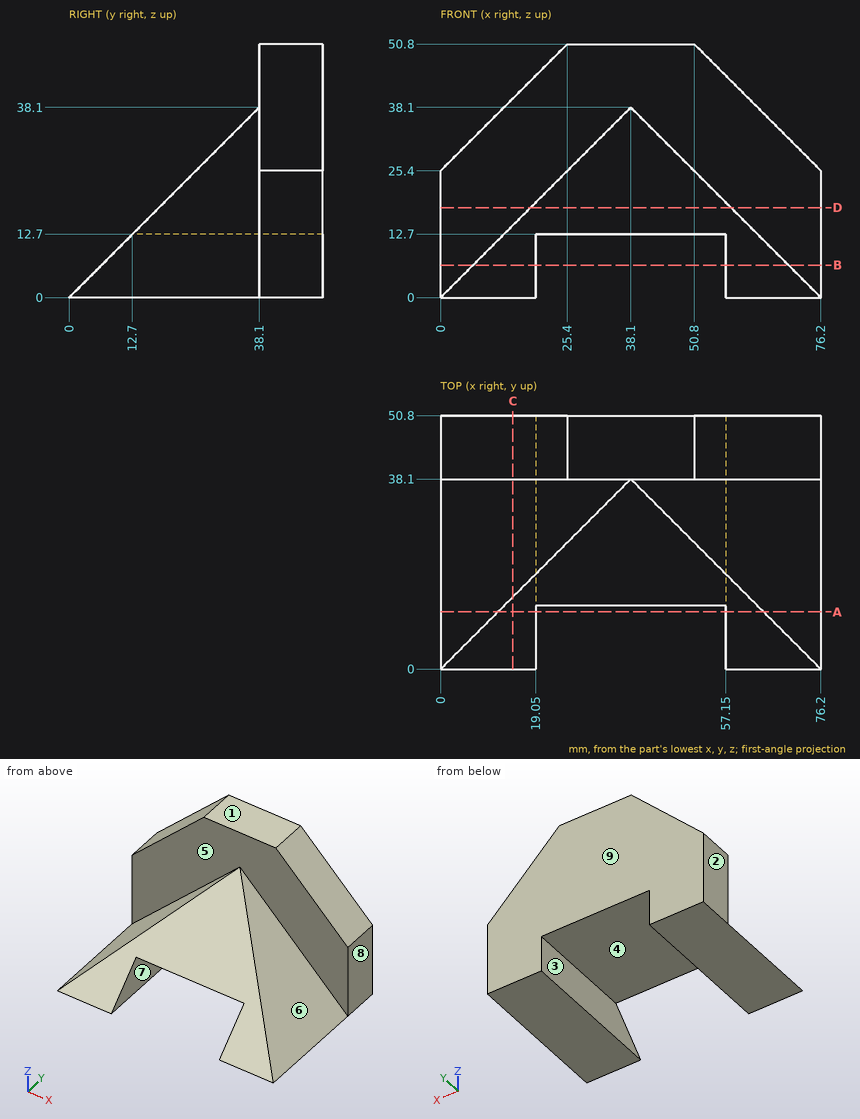
Geometry check sheet. Reference: drawing and pictorial views, mm from the part's lowest x, y, z. A direction names the side the tool comes from. Give positions to 0.01 mm unless a question says otherwise; leave off trailing zeros. Loops run counter-clockwise (first coordinate to the right, second up) from the corner with the lowest first, then second, coordinate; pieces in that order, holes last. Notation, with made-up numbers: (-4, 27.5) - (25, 27.5) arc R6 ccw to (25, 33.5) - close; hole circle Ø2 at (37.5, -19). An arc over 180 degrees is marked (long way). One line per question, with ' | ' between items. Start each with the question number.
1. Draft check along X on the marked faces 1, 2, 3 and 4. Enter one of: released by +X, released by -X, zero draft, split by the parting line, or undercut.
2. Cross-section at B-B, the plane z = 6.5. Enter the section's corners in (x, y).
3. Cross-section at D-D, the plane z = 18. Enter the section's corners in (x, y), plus the area to 3 significant figures.
4. Material ranges on line 1 along Y through (x, z) = (39, 45); line 2 along X through (y, z) = (8, 3.5); line 3 along X through (y, z) = (28.5, 6.5), recorded low to high. Write a range as [from, to].
5. Cross-section at C-C, the plane x = 14.5. Enter the section's corners in (y, z), plus the area to 3 significant figures.
6. Gauge pin test, flat ends, axial feed: pin 1 Ø11.5 at (x, y) = (31, 23.5) entering from -Z; pin 2 Ø2 at (y, z) = (36, 43.5) entering from -X; pin 3 Ø10 at (y, z) = (23.5, 9) entering from -X; pin 4 Ø3 at (x, y) = (49.5, 12.5) entering from +Z. Record the tip position at first contact, or that the pin passes through.
7. Cross-section at A-A, the plane y = 11.5. Enter the section's corners in (x, z), plus the area to 3 significant figures.
8. Set-up check for the marked faces 5, 6, 7, 8 and 9: record each of +Z, -Z, +X, -X, +Y, -Y from which the full face is reachable in a straight line by a thin tool's end or side.
Check result:
1) face 1: zero draft | face 2: released by -X | face 3: undercut | face 4: undercut
2) outline: (0, 38.1) - (6.5, 38.1) - (6.5, 6.5) - (19.05, 6.5) - (19.05, 50.8) - (0, 50.8) - close; (57.15, 6.5) - (69.7, 6.5) - (69.7, 38.1) - (76.2, 38.1) - (76.2, 50.8) - (57.15, 50.8) - close
3) outline: (0, 38.1) - (18, 38.1) - (18, 18) - (58.2, 18) - (58.2, 38.1) - (76.2, 38.1) - (76.2, 50.8) - (0, 50.8) - close | area: 1,780 mm2
4) line 1: y = [38.1, 50.8] | line 2: x = [3.5, 19.05], [57.15, 72.7] | line 3: x = [6.5, 19.05], [57.15, 69.7]
5) outline: (0, 0) - (50.8, 0) - (50.8, 39.9) - (38.1, 39.9) - (38.1, 14.5) - (14.5, 14.5) - close | area: 954 mm2
6) pin 1: stops at z = 12.7 | pin 2: passes through | pin 3: stops at x = 4 | pin 4: stops at z = 14
7) outline: (0, 0) - (19.05, 0) - (19.05, 11.5) - (11.5, 11.5) - close; (57.15, 0) - (76.2, 0) - (64.7, 11.5) - (57.15, 11.5) - close | area: 306 mm2
8) face 5: +Z, -Y | face 6: +Z, +X, -Y | face 7: -Z, +Y, -Y | face 8: +Z, -Z, +X, +Y, -Y | face 9: +Z, -Z, +X, -X, +Y
